Verification items for the finished model (mm, model axes). A direction names the side the tool comes from. Give positions to 0.01 mm unless a question says otherwise; leave off trailing zeros. Loops run counter-clockwise (first coordinate to the right, second up) from the corner with the lowest first, then second, coordinate; pieces in that order, holes last. Notation, with made-up numbers: M 84.5,73 L 101.5,73 A22 cw 101.5,89 Z; hole C 87,63.5 d8. An arc over 180 degrees is marked long. Put each result on its own line as item: value. Start each with the question number.
Autodesk Inventor part; units mm, degrees
ref_plane "YZ Plane" through (0, 0, 0) normal (1, 0, 0) x (0, 1, 0)
ref_plane "XZ Plane" through (0, 0, 0) normal (0, 1, 0) x (-1, 0, 0)
ref_plane "XY Plane" through (0, 0, 0) normal (0, 0, 1) x (1, 0, 0)
sketch "Skizze1" plane through (0, 0, 0) normal (0, 0, 1) x (1, 0, 0)
  circle A0 centre (0, 0) radius 16
  circle A1 centre (-8, 8) radius 2
  line L0 (0, 16) -> (0, -16) construction
  line L1 (-16, 0) -> (16, 0) construction
  circle A2 centre (8, 8) radius 2
  circle A3 centre (-8, -8) radius 2
  circle A4 centre (8, -8) radius 2
  circle A5 centre (0, 0) radius 5
  circle A6 centre (0, 0) radius 3
  dimension "d0" = 32
  dimension "d1" = 4
  dimension "d2" = 8
  dimension "d3" = 8
  dimension "d6" = 16
  dimension "d9" = 16
  dimension "d16" = 10
  dimension "d19" = 6
extrude "Extrusion1" add sketch "Skizze1" along normal mid plane 57.2 contours A0 | A1 | A2 | A3 | A4 | A5 | A6
extrude "Extrusion2" cut sketch "Skizze1" against normal blind 10 from surface at 28.6 contours A1 | A2 | A3 | A4
extrude "Extrusion3" add sketch "Skizze1" along normal blind 1 from surface at 28.6 contours A5 | A6
extrude "Extrusion4" cut sketch "Skizze1" along normal through all both and the other way through all contours A6
mirror "Spiegeln1" about plane through (0, 0, 0) normal (0, 0, 1) of "Extrusion2"
equation "\"d2\" = Montage"
equation "\"d3\" = Montage"
equation "\"d6\" = 2 * Montage"
equation "\"d9\" = 2 * Montage"
equation "\"Montage\" = 8"
properties part number "Generator" material "ABS-Kunststoff"
Q1. Cross-section at A-A, the plane x = 0. Record the boundary of the cut face in (y, z), then the cut area to 3 significant figures.
Q2. Set-up check for faces 1 (the face through (6, 8, -24)), 2 (the face through (-3, 0, 1)), 3 (the face through (-9.474, 9.352, 23.67)): record each of +Z, -Z, +X, -X, +Y, -Y from which the full face is reachable in a straight line by a thin tool's end or side.
Q3. Go/stop test with flat-tipped pins: pin 1 (4.5 mm diameter, centred on x = -7.5, y = -9, fed in from +Z); pin 2 (1.2 mm diameter, centred on x = -7, y = 7.5, fed in from -Z); pin 3 (2.5 mm diameter, centred on x = 8, y = -8, fed in from +Z). Record where each tip stops, or that it passes through.
Q4. Cross-section at D-D, the plane x = 8. Record the boundary of the cut face in (y, z), then the cut area to 3 significant figures.
Q5. Cross-section at C-C, the plane z = 0. Record the boundary of the cut face in (x, y), then the cut area to 3 significant figures.
Q6. Scan lines: L1, parallel to Y at x = 0, z = 5; L2, parallel to Z at x = -5.5, y = -2; L3, parallel to Y at x = -8, z = -20.25. Record each from-to range of solid material in increasing order.
Q7. Release check for a two-part mould opening along X. For faces 4 (the face through (-0.2, -3.3, -28.6)), 5 (the face through (-3.47, -15.62, 0.4)), 6 (the face through (6.526, -9.352, -23.67)) record: pulls with the +X half, pulls with the -X half, needs draft (parallel to the pull), parting line crosses it, or undercut.
Ans:
1. outline: M -16,-28.6 L -3,-28.6 L -3,29.6 L -5,29.6 L -5,28.6 L -16,28.6 Z; M 3,-28.6 L 16,-28.6 L 16,28.6 L 5,28.6 L 5,29.6 L 3,29.6 Z
1. area: 1,490 mm^2
2. face 1: -Z
2. face 2: +Z, -Z
2. face 3: +Z
3. pin 1: stops at z = 28.6
3. pin 2: stops at z = -18.6
3. pin 3: stops at z = 18.6
4. outline: M -13.86,-28.6 L -10,-28.6 L -10,-18.6 L -6,-18.6 L -6,-28.6 L 6,-28.6 L 6,-18.6 L 10,-18.6 L 10,-28.6 L 13.86,-28.6 L 13.86,28.6 L 10,28.6 L 10,18.6 L 6,18.6 L 6,28.6 L -6,28.6 L -6,18.6 L -10,18.6 L -10,28.6 L -13.86,28.6 Z
4. area: 1,430 mm^2
5. outline: C 0,0 d32; hole C 0,0 d6
5. area: 776 mm^2
6. L1: y = -16 to -3, 3 to 16
6. L2: z = -28.6 to 28.6
6. L3: y = -13.86 to -10, -6 to 6, 10 to 13.86
7. face 4: needs draft
7. face 5: parting line crosses it
7. face 6: undercut
